Could you check a few things on this model? Use its own coordinates, in mm. Face numbers are marked on the shaded views. A direction names the side the tool comes from. Coordinates: 2 decimals unless noted, no trailing zeros. Loops run counter-clockwise (first coordinate to the right, second up) from the corner with the lowest first, then second, coordinate; pieces in that order, holes last.
from build123d import *

# Parameters (mm, degrees)
F2_DEPTH = 10
F3_W     = 60
F3_H     = 10
F3_W_2   = 10
F3_H_2   = 60
F4_DEPTH = 60
F5_R     = 4.99999


# Not quite as in the source:
# - a fillet or chamfer is up to 0.001 mm smaller than in the source, because OpenCascade refuses the exact size


with BuildPart() as f2:
    # F1 (on Top) → F2 (new body)
    with BuildSketch(Plane.XY):
        Polygon((-11, 65.8), (-11, -11), (49, -11), (49, 25.8), (143.4, 25.8), (143.4, 85.8), (96, 85.8), (96, 65.8), align=None)
    extrude(amount=F2_DEPTH)

    # F3 (on face) → F4 (join)
    with BuildSketch(Plane(origin=(0, 0, 0), x_dir=(1, 0, 0), z_dir=(0, 0, -1))):
        with Locations((19, 6)):
            Rectangle(F3_W, F3_H)
        with Locations((19, -24.5)):
            Rectangle(F3_W, F3_H)
        with Locations((101, -55.8)):
            Rectangle(F3_W_2, F3_H_2)
        with Locations((138.4, -55.8)):
            Rectangle(F3_W_2, F3_H_2)
    extrude(amount=F4_DEPTH)

    # F5 (radius 5 in the source; OpenCascade refuses exactly that, so slightly less here)
    f5_edges = [f2.edges().sort_by_distance(p)[0] for p in [
        (96, 65.8, 5),
        (96, 85.8, -25),
        (143.4, 85.8, -25),
        (-11, 65.8, 5),
        (-11, 29.5, -30),
        (-11, -11, -25),
        (119.7, 85.8, 0),
        (42.5, 65.8, 0),
        (-11, 47.65, 0),
        (-11, 9.25, 0),
        (133.4, 55.8, -60),
        (106, 55.8, -60),
        (96, 55.8, -60),
        (143.4, 55.8, -60),
        (19, 29.5, 0),
        (19, 29.5, -60),
        (19, -11, -60),
        (19, -1, -60),
        (19, 19.5, -60),
        (96, 45.8, 0),
    ]]
    fillet(f5_edges, radius=F5_R)


solid = f2.part
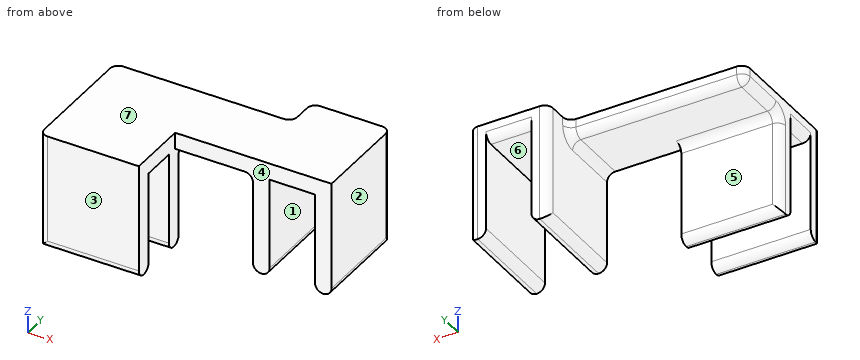
(1) Imagine slicing it at A-A, the plane z = -29. Write out the boundary of the cut face in (x, y), and give its area (3 significant figures).
Answers:
outline: (-11, -6) arc R5 ccw to (-6, -11) - (49, -11) - (49, -1) - (-11, -1) - close; (-11, 19.5) - (49, 19.5) - (49, 29.5) - (-6, 29.5) arc R5 ccw to (-11, 24.5) - close; (96, 25.8) - (106, 25.8) - (106, 85.8) - (101, 85.8) arc R5 ccw to (96, 80.8) - close; (133.4, 25.8) - (143.4, 25.8) - (143.4, 80.8) arc R5 ccw to (138.4, 85.8) - (133.4, 85.8) - close
area: 2,380 mm2
(2) Which directions (+Z, -Z, +X, -X, +Y, -Y) give clear straight access to the entire face, cutting with the end or side of a thin tool? Please do the marked faces 4, 5, 6 and 7.
Answers:
face 4: +Z, -Z, +X, -Y
face 5: -Z, -X, +Y
face 6: -Z, +Y, -Y
face 7: +Z, +X, -X, +Y, -Y
(3) We'd pull the mould along X, two halves only. Please class the marked faces 1, 2 and 3: +X half, -X half, draft (parallel to the pull), parting line (faces both ways), or undercut.
Answers:
face 1: undercut
face 2: +X half
face 3: draft
(4) For pin 1 (8 mm diameter, centred on y = 57, z = -50.5, fed in from -X); pin 2 (13.5 mm diameter, centred on y = 22.5, z = -10.5, fed in from +X); pin 3 (4 mm diameter, centred on x = 65, z = 7, fed in from +Y); pin 4 (18 mm diameter, centred on x = 20, z = -14.5, fed in from +Y), each with a flat end and sliding along its axis, tell me the tip position at first contact or that it passes through.
Answers:
pin 1: stops at x = 96
pin 2: stops at x = 143.4
pin 3: stops at y = 65.8
pin 4: stops at y = 29.5
(5) I need wall thicknesses on probe 1 along Y at (x, z) = (39.5, -5); probe 2 along X at (y, z) = (79, -33.5); probe 3 along Z at (x, y) = (44, -0.5). Which ranges of each line are inside material? Lowest first, please.
Answers:
probe 1: y = -11 to -1, 19.5 to 29.5
probe 2: x = 96 to 106, 133.4 to 143.4
probe 3: z = 0 to 10
